The listing builds one solid part. Answer for the finished solid, in the listing's coordinates (mm). Face numbers are marked on the shaded views. Round coordinates to 2 decimals unless told otherwise and drop trailing zeros. Order: outer loops, then holes, each group sorted by start corner. A loop starts at its lowest first (then second) coordinate and runs counter-clockwise, first axis right, second up. Notation, with made-up numbers: (15.5, 27.25) - (71.5, 27.25) arc R4 cw to (71.5, 33.25) - close; hole circle Ø8 at (63, 74.5). An arc over 180 degrees is marked (long way). One line per item, written item: value. Start each with the question number.
1. For a pull along Z with two mould halves and no side action, classify the marked faces 1 and 2 as released by +Z, released by -Z, zero draft, split by the parting line, or undercut.
2. Straight lines are drawn through the part: line 1 (X direction, y = -3.5, z = 38.5); line 2 (X direction, y = -6.75, z = -55); line 3 (Y direction, x = -24.5, z = -39). For each, find the intervals that lie inside material, in ascending order.
3. Section B-B, the plane x = -18 is taken. Give the vertices of the cut face in (y, z), then the cut area to 3 significant figures.
4. Section A-A, the plane z = -50 is taken. Give the vertices of the cut face in (x, y), then the cut area to 3 significant figures.
5. Flat-ended cylindrical pins translate along their axes: P1, Ø1.5, axis at x = 16.5, z = 26.5, coming from the +Y side; P2, Ø1.3, axis at x = -15, y = -3.5, coming from the +Z side. Find the tip coordinate at first contact, or state that the pin passes through.
from build123d import *

# Parameters (mm, degrees)
F0_W     = 78.0542
F0_H     = 127
F1_DEPTH = 10.16
F2_T     = -7.62
F3_T     = -2.54


with BuildPart() as f1:
    # F0 (on Front) → F1 (new body)
    with BuildSketch(Plane.XZ):
        Rectangle(F0_W, F0_H)
    extrude(amount=F1_DEPTH)

    # F2
    f2_openings = [f1.faces().sort_by_distance(p)[0] for p in [
        (0, 0, 0),
    ]]
    offset(amount=F2_T, openings=f2_openings)

    # F3
    f3_openings = [f1.faces().sort_by_distance(p)[0] for p in [
        (0, -5.08, 63.5),
    ]]
    offset(amount=F3_T, openings=f3_openings, kind=Kind.INTERSECTION)


solid = f1.part
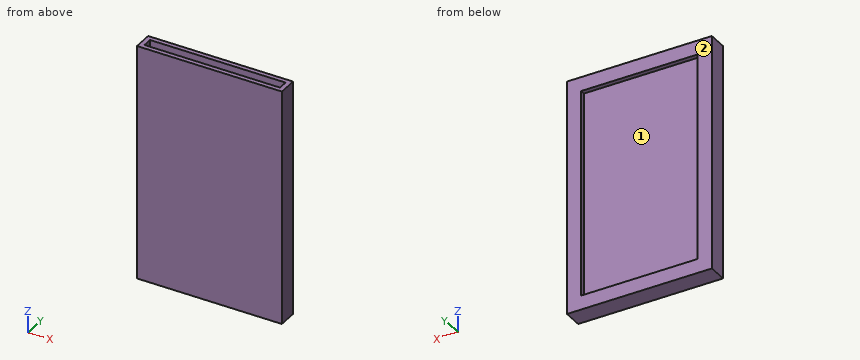
Answer list:
1. face 1: undercut
1. face 2: zero draft
2. line 1: x = -39.03 to -36.49, -33.95 to 33.95, 36.49 to 39.03
2. line 2: x = -39.03 to -36.49, 36.49 to 39.03
2. line 3: y = -10.16 to -7.62, -5.08 to -2.54
3. outline: (-10.16, -63.5) - (0, -63.5) - (0, -55.88) - (-2.54, -55.88) - (-2.54, 55.88) - (0, 55.88) - (0, 63.5) - (-2.54, 63.5) - (-2.54, 58.42) - (-5.08, 58.42) - (-5.08, -58.42) - (-2.54, -58.42) - (-2.54, -60.96) - (-7.62, -60.96) - (-7.62, 63.5) - (-10.16, 63.5) - close
3. area: 671 mm²
4. outline: (-39.03, -10.16) - (39.03, -10.16) - (39.03, 0) - (31.41, 0) - (31.41, -2.54) - (-31.41, -2.54) - (-31.41, 0) - (-39.03, 0) - close; hole (-36.49, -7.62) - (36.49, -7.62) - (36.49, -2.54) - (33.95, -2.54) - (33.95, -5.08) - (-33.95, -5.08) - (-33.95, -2.54) - (-36.49, -2.54) - close
4. area: 435 mm²
5. P1: stops at y = -2.54
5. P2: stops at z = 58.42
